Here's the drawing with two shaded views (mm, measured from the low corner). I have some questions. A direction names the side the tool comes from. Give positions to 0.01 mm unless a question says otherwise; leave off trailing zeros. Loops run counter-clockwise (first coordinate to the right, second up) from the corner with the lowest first, then second, coordinate; pieces in that order, holes last. Notation, with made-up numbers: M 40,11.25 L 96,11.25 A22 ccw 96,23.25 Z; hole C -15.75,-7.5 d6. An arc over 180 degrees is marked long. Use a Markdown table: item, result. Add a question column.
1) If I drill on line 1 along X through (y, z) = (65.5, 42.5); line 2 along Z through (x, y) = (18.5, 28); line 3 along Z through (x, y) = (27, 55), over which ranges is the centre line in solid material (lowest first)? Write a range as [from, to].
2) Will these pins go through, and if not, where does the flat tip stop? pin 1 Ø2.5 at (x, z) = (48.5, 5) entering from -Y; pin 2 Ø22 at (x, z) = (32.5, 7.5) entering from -Y; pin 3 Ø8 at (x, y) = (8.5, 18) entering from +Z.
3) Suppose I cut it at D-D on y = 62. List the corners of the cut face in (x, z) for me.
4) Suppose I cut it at A-A on y = 16. List the corners of the cut face in (x, z) for me.
5) Suppose I cut it at B-B on z = 17. List the corners of the cut face in (x, y) for me, and give its area (3 significant figures).
6) Suppose I cut it at C-C on x = 29.5. List the corners of the cut face in (y, z) for me.
7) We'd pull the mould along X, two halves only. Please class the marked faces 1, 2 and 3: +X half, -X half, draft (parallel to the pull), parting line (faces both ways), or undercut.
8) Which directions (+Z, -Z, +X, -X, +Y, -Y) give clear straight access to the entire face, cutting with the end or side of a thin tool? Please do the marked faces 4, 5, 6 and 7.
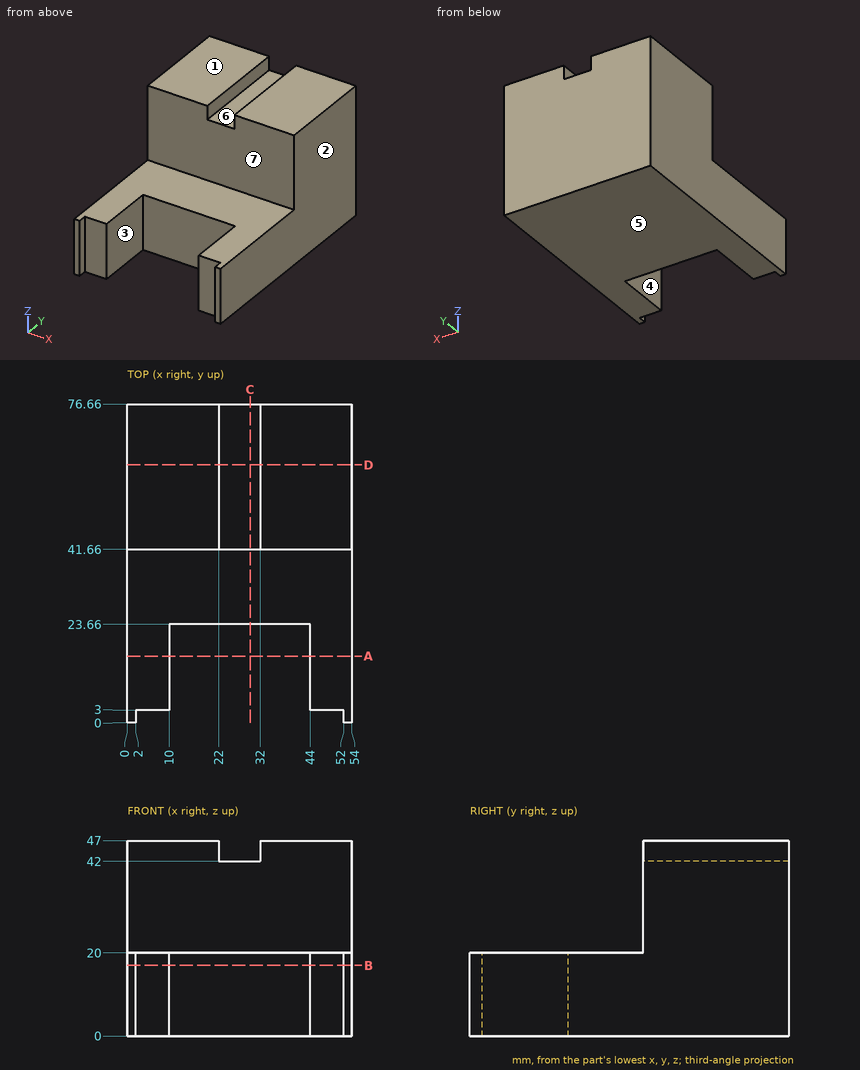
Answer block:
| question | item | result |
|---|---|---|
| 1 | line 1 | x = [0, 22], [32, 54] |
| 1 | line 2 | z = [0, 20] |
| 1 | line 3 | z = [0, 42] |
| 2 | pin 1 | stops at y = 3 |
| 2 | pin 2 | stops at y = 23.66 |
| 2 | pin 3 | stops at z = 20 |
| 3 | outline | M 0,0 L 54,0 L 54,47 L 32,47 L 32,42 L 22,42 L 22,47 L 0,47 Z |
| 4 | outline | M 0,0 L 10,0 L 10,20 L 0,20 Z; M 44,0 L 54,0 L 54,20 L 44,20 Z |
| 5 | outline | M 0,0 L 2,0 L 2,3 L 10,3 L 10,23.66 L 44,23.66 L 44,3 L 52,3 L 52,0 L 54,0 L 54,76.66 L 0,76.66 Z |
| 5 | area | 3,290 mm^2 |
| 6 | outline | M 23.66,0 L 76.66,0 L 76.66,42 L 41.66,42 L 41.66,20 L 23.66,20 Z |
| 7 | face 1 | draft |
| 7 | face 2 | +X half |
| 7 | face 3 | undercut |
| 8 | face 4 | +Z, -Z, -Y |
| 8 | face 5 | -Z, +X, -X, +Y, -Y |
| 8 | face 6 | +Z, +Y, -Y |
| 8 | face 7 | +Z, +X, -X, -Y |
